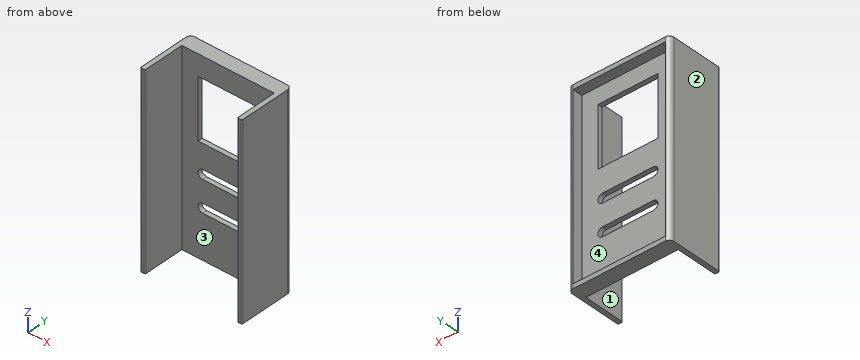
from build123d import *

# Parameters (mm, degrees)
BOSS_EXTRUDE1_DEPTH = 410
SKETCH4_W           = 200
SKETCH4_H           = 390
CUT_EXTRUDE1_DEPTH  = 21.5
SKETCH5_W           = 130
SKETCH5_H           = 130
CUT_EXTRUDE2_DEPTH  = 30
SKETCH9_W           = 10
SKETCH9_H           = 410
BOSS_EXTRUDE2_DEPTH = 2
SKETCH10_W          = 10
SKETCH10_H          = 410
BOSS_EXTRUDE3_DEPTH = 2
CUT_EXTRUDE4_DEPTH  = 600


with BuildPart() as part:
    # Sketch3 → Boss-Extrude1 (new body)
    with BuildSketch(Plane.XY):
        Polygon((-76.099744246, 40.652173913), (143.900255754, 40.652173913), (143.900255754, -79.347826087), (133.900255754, -79.347826087), (133.900255754, 9.152173913), (-66.099744246, 9.152173913), (-66.099744246, -79.347826087), (-76.099744246, -79.347826087), align=None)
    extrude(amount=-BOSS_EXTRUDE1_DEPTH)

    # Sketch4 → Cut-Extrude1 (cut)
    with BuildSketch(Plane(origin=(0, 40.652173913, 0), x_dir=(1, 0, 0), z_dir=(0, 1, 0))):
        with Locations((33.900255754, 205)):
            Rectangle(SKETCH4_W, SKETCH4_H)
    extrude(amount=-CUT_EXTRUDE1_DEPTH, mode=Mode.SUBTRACT)

    # Sketch5 → Cut-Extrude2 (cut)
    with BuildSketch(Plane(origin=(0, 19.152173913, 0), x_dir=(1, 0, 0), z_dir=(0, 1, 0))):
        with Locations((33.900255754, 110)):
            Rectangle(SKETCH5_W, SKETCH5_H)
        with BuildLine():
            Line((-21.099744246, 247.552781264), (88.900255754, 247.552781264))
            ThreePointArc((88.900255754, 247.552781264), (98.900255754, 237.552781264), (88.900255754, 227.552781264))
            Line((88.900255754, 227.552781264), (-21.099744246, 227.552781264))
            ThreePointArc((-21.099744246, 227.552781264), (-31.099744246, 237.552781264), (-21.099744246, 247.552781264))
        make_face()
        with BuildLine():
            Line((-21.099744246, 315.266550997), (88.900255754, 315.266550997))
            ThreePointArc((88.900255754, 315.266550997), (98.900255754, 305.266550997), (88.900255754, 295.266550997))
            Line((88.900255754, 295.266550997), (-21.099744246, 295.266550997))
            ThreePointArc((-21.099744246, 295.266550997), (-31.099744246, 305.266550997), (-21.099744246, 315.266550997))
        make_face()
    extrude(amount=-CUT_EXTRUDE2_DEPTH, mode=Mode.SUBTRACT)

    # Sketch9 → Boss-Extrude2 (add)
    with BuildSketch(Plane.XZ.offset(79.347826087)):
        with Locations((138.900255754, -205)):
            Rectangle(SKETCH9_W, SKETCH9_H)
    extrude(amount=BOSS_EXTRUDE2_DEPTH)

    # Sketch10 → Boss-Extrude3 (add)
    with BuildSketch(Plane.XZ.offset(79.347826087)):
        with Locations((-71.099744246, -205)):
            Rectangle(SKETCH10_W, SKETCH10_H)
    extrude(amount=BOSS_EXTRUDE3_DEPTH)

    # Sketch11 → Cut-Extrude4 (cut)
    with BuildSketch(Plane.XY):
        with BuildLine():
            Line((-76.099744246, 40.652173913), (-76.099744246, 30.652173913))
            ThreePointArc((-76.099744246, 30.652173913), (-73.170812057, 37.723241725), (-66.099744246, 40.652173913))
            Line((-66.099744246, 40.652173913), (-76.099744246, 40.652173913))
        make_face()
        with BuildLine():
            Line((143.900255754, 40.652173913), (133.900255754, 40.652173913))
            ThreePointArc((133.900255754, 40.652173913), (140.971323566, 37.723241725), (143.900255754, 30.652173913))
            Line((143.900255754, 30.652173913), (143.900255754, 40.652173913))
        make_face()
        with BuildLine():
            Line((143.900255754, -81.347826087), (143.900255754, -79.347826087))
            ThreePointArc((143.900255754, -79.347826087), (143.314469317, -80.762039649), (141.900255754, -81.347826087))
            Line((141.900255754, -81.347826087), (143.900255754, -81.347826087))
        make_face()
        with BuildLine():
            Line((133.900255754, -81.347826087), (135.900255754, -81.347826087))
            ThreePointArc((135.900255754, -81.347826087), (134.486042192, -80.762039649), (133.900255754, -79.347826087))
            Line((133.900255754, -79.347826087), (133.900255754, -81.347826087))
        make_face()
        with BuildLine():
            ThreePointArc((-74.099744246, -81.347826087), (-75.513957808, -80.762039649), (-76.099744246, -79.347826087))
            Line((-76.099744246, -79.347826087), (-76.099744246, -81.347826087))
            Line((-76.099744246, -81.347826087), (-74.099744246, -81.347826087))
        make_face()
        with BuildLine():
            ThreePointArc((-66.099744246, -79.347826087), (-66.685530683, -80.762039649), (-68.099744246, -81.347826087))
            Line((-68.099744246, -81.347826087), (-66.099744246, -81.347826087))
            Line((-66.099744246, -81.347826087), (-66.099744246, -79.347826087))
        make_face()
    extrude(amount=-CUT_EXTRUDE4_DEPTH, mode=Mode.SUBTRACT)


solid = part.part
CAD build for the part. Positions are in the model's coordinates, mm. Face numbers are marked on the shaded views. A direction names the side the tool comes from. Give positions to 0.01 mm unless a question says otherwise; leave off trailing zeros. Loops run counter-clockwise (first coordinate to the right, second up) from the corner with the lowest first, then second, coordinate; pieces in that order, holes last. Notation, with made-up numbers: M -12.75,22.25 L 11.25,22.25 A21 cw 11.25,41.25 Z; hole C 8.5,61.5 d1. An arc over 180 degrees is marked long. One line per question, with ' | ' between items. Start each with the question number.
1. Saw through at A-A on y = -53.5. Give the cut face in (x, z), plus the area to 3 significant figures.
2. Saw through at C-C on x = 52. Give the cut face in (y, z), plus the area to 3 significant figures.
3. Saw through at D-D on x = -38. Give the cut face in (y, z).
4. Two-plate mould, pull along Z, no slides. Class the marked faces 3 and 4: pulls with the +Z half, pulls with the -Z half, needs draft (parallel to the pull), parting line crosses it, or undercut.
5. Probe L1, parallel to Z at x = 65.5, y = 12; L2, parallel to X at y = 21.5, z = -224.5; L3, parallel to Z at x = 85, y = 26. List the from-to ranges inside material, lowest first. Write a range as from..to.
6. Saw through at B-B on z = -128.5. Give the cut face in (x, y).
7. 3-axis set-ups, long thin cutter, end or side, ignore diameter. For the marked faces 1 and 2: which of +Z, -Z, +X, -X, +Y, -Y reach the whole face in a straight line?
Result sheet:
1) outline: M -76.1,-410 L -66.1,-410 L -66.1,0 L -76.1,0 Z; M 133.9,-410 L 143.9,-410 L 143.9,0 L 133.9,0 Z | area: 8,200 mm^2
2) outline: M 9.15,-410 L 40.65,-410 L 40.65,-400 L 19.15,-400 L 19.15,-315.27 L 9.15,-315.27 Z; M 9.15,-295.27 L 19.15,-295.27 L 19.15,-247.55 L 9.15,-247.55 Z; M 9.15,-227.55 L 19.15,-227.55 L 19.15,-175 L 9.15,-175 Z; M 9.15,-45 L 19.15,-45 L 19.15,-10 L 40.65,-10 L 40.65,0 L 9.15,0 Z | area: 2,830 mm^2
3) outline: M 9.15,-410 L 40.65,-410 L 40.65,-400 L 19.15,-400 L 19.15,-10 L 40.65,-10 L 40.65,0 L 9.15,0 Z
4) face 3: needs draft | face 4: undercut
5) L1: z = -410..-315.27, -295.27..-247.55, -227.55..-175, -45..0 | L2: x = -76.1..-66.1, 133.9..143.9 | L3: z = -410..-400, -10..0
6) outline: M -76.1,-79.35 A2 ccw -74.1,-81.35 L -68.1,-81.35 A2 ccw -66.1,-79.35 L -66.1,9.15 L -31.1,9.15 L -31.1,19.15 L -66.1,19.15 L -66.1,40.65 A10 ccw -76.1,30.65 Z; M 98.9,9.15 L 133.9,9.15 L 133.9,-79.35 A2 ccw 135.9,-81.35 L 141.9,-81.35 A2 ccw 143.9,-79.35 L 143.9,30.65 A10 ccw 133.9,40.65 L 133.9,19.15 L 98.9,19.15 Z
7) face 1: +Z, -Z, -Y | face 2: +Z, -Z, -X, +Y, -Y
